Solid Edge part; units mm, degrees
sketch "Sketch1" plane through (0, 0, 0) normal (0, -1, 0) x (1, 0, 0)
  circle A0 centre (0, 0) radius 50
extrude "Protrusion1" add sketch "Sketch1" along normal mid plane 25
sketch "Sketch2" plane through (0, 0, 0) normal (1, 0, 0) x (0, 1, 0)
  circle A0 centre (0, 65) radius 17.5
revolve "RevolvedCutout1" cut sketch "Sketch2" angle 360 about axis through (0, -60, 0) along (0, 1, 0)
sketch "Sketch3" plane through (0, -12.5, 0) normal (0, -1, 0) x (1, 0, 0)
  circle A0 centre (0, 0) radius 15
extrude "Cutout1" cut sketch "Sketch3" against normal up to next
sketch "Sketch4" plane through (0, 0, 0) normal (1, 0, 0) x (0, 1, 0)
  line L0 (-12.5, 45) -> (-9.0139, 50)
revolve "RevolvedCutout2" cut sketch "Sketch4" angle 360 about axis through (0, -60, 0) along (0, 1, 0) material side at (0, -10.798, 47.5286)
mirror "Mirror1" about plane through (0, 0, 0) normal (0, -1, 0) of "RevolvedCutout2"
properties material "Steel"
Input: part model. Units: mm. Frame: model coordinates. Give positions to 0.01 mm unless a question says otherwise; leave off trailing zeros. Loops run counter-clockwise (first coordinate to the right, second up) from the corner with the lowest first, then second, coordinate; pieces in that order, holes last. Notation, with made-up numbers: M 2,46.5 L 20,46.5 A25 ccw 20,61.5 Z; hole C 64,10 d8. An arc over 180 degrees is marked long. Answer as CSV lines item,"result". Start each with the question number.
1. Pin query (flat end, axial travel): P1, Ø3, axis at y = -4, z = 16.5, coming from the -X side; P2, Ø12, axis at y = 0.5, z = 24.5, coming from the +X side; P3, Ø3, axis at x = -8.5, y = 7, coming from the -Z side. Return the tip coordinate at first contact, or that it passes through.
2. Section C-C on y = 11.25. Return loops of the section in (x, z), plus the area to 3 significant figures.
3. Section D-D on y = -2.5. Return loops of the section in (x, z), plus the area to 3 significant figures.
4. Line query: L1, parallel to Z at x = 0, y = -6; L2, parallel to Z at x = 0, y = -3.25; L3, parallel to Z at x = 17.5, y = 2. Output: solid intervals per line, ascending.
5. Pull-direction query (X, two-part tool) for faces 1 (the face through (30.625, -12.282, -33.397)), 2 (the face through (-14.985, -0.175, 0.66)), 3 (the face through (11, -12.5, 11)); classes: released by +X, released by -X, zero draft, split by the parting line, or undercut.
Computed values:
1,P1,"stops at x = -45.71"
1,P2,"stops at x = 43.8"
1,P3,"stops at z = -49.01"
2,outline,"C 0,0 d93.59; hole C 0,0 d30"
2,area,"6,170 mm²"
3,outline,"C 0,0 d95.36; hole C 0,0 d30"
3,area,"6,440 mm²"
4,L1,"z = -48.56 to -15, 15 to 48.56"
4,L2,"z = -47.8 to -15, 15 to 47.8"
4,L3,"z = -44.28 to 44.28"
5,face 1,"split by the parting line"
5,face 2,"undercut"
5,face 3,"zero draft"
